Work out the finished part from the listing and answer in its coordinate system (mm). A direction names the side the tool comes from. Coordinates: 2 decimals unless noted, no trailing zeros. Order: outer loops, then holes, each group sorted by start corner. A loop starts at its lowest first (then second) coordinate and runs counter-clockwise, first axis right, second up.
Autodesk Inventor part; units mm, degrees
ref_plane "YZ Plane" through (0, 0, 0) normal (1, 0, 0) x (0, 1, 0)
ref_plane "XZ Plane" through (0, 0, 0) normal (0, 1, 0) x (-1, 0, 0)
ref_plane "XY Plane" through (0, 0, 0) normal (0, 0, 1) x (1, 0, 0)
sketch "Sketch1" plane through (0, 0, 0) normal (1, 0, 0) x (0, 1, 0)
  line L0 (0, 15) -> (2.5, 15) construction
  line L1 (0, 0) -> (9.4946, 0) construction
  arc A0 (9.4946, 0) -> (2.5, 15) centre (-10.0865, 0) ccw construction
  line L2 (0, 9.5) -> (0, 0) construction
  line L3 (9.4946, 0) -> (9, 0) construction
  line L4 (9, 0) -> (9, 15)
  line L5 (9, 15) -> (9, 15)
  line L6 (9, 15) -> (9, 17)
  line L7 (9, 17) -> (4.25, 17)
  line L8 (4.25, 17) -> (4.25, 15)
  line L9 (2.5, 15) -> (4.25, 15) construction
  line L10 (2.5, 15) -> (9.4946, 0) construction
  line L11 (3.25, 15) -> (3.25, 13.3916)
  line L12 (3.25, 15) -> (4.25, 15)
  line L13 (7.1631, 5) -> (7.1631, 0)
  line L14 (7.1631, 0) -> (9, 0)
  line L15 (7.1631, 5) -> (3.25, 13.3916)
  point P0 (2.25, 0)
  dimension "d2" = 15
  dimension "d12" = 2
  dimension "d14" = 0
  dimension "d16" = 2
  dimension "d17" = 4.25
  dimension "d35" = 115
  dimension "d36" = 9
  dimension "d37" = 2.5
  dimension "d39" = 1
  dimension "d40" = 5
  dimension "d41" = 7.1631
  dimension "d42" = 3.25
  dimension "d43" = 1.6084
  dimension "d44" = 8.3916
revolve "Revolution1" add sketch "Sketch1" angle 360 about axis through (0, 0, 9.5) along (0, 0, -1)
sketch "Sketch3" plane through (0, 0, 0) normal (1, 0, 0) x (0, 1, 0)
  line L0 (7.1631, 0) -> (14, 0)
  line L1 (14, 0) -> (14, 17)
  line L2 (14, 17) -> (7.1631, 17)
  line L3 (7.1631, 17) -> (7.1631, 0)
  line L4 (-7.1631, 0) -> (7.1631, 0) construction
  line L5 (-9, 17) -> (9, 17) construction
  point P0 (0, 0)
  dimension "d28" = 14
extrude "Extrusion1" add sketch "Sketch3" along normal mid plane 8
sketch "Sketch4" plane through (-4, 0, 0) normal (-1, 0, 0) x (0, 0, 1)
  circle A0 centre (5, 10.25) radius 1.6
  circle A1 centre (12, 10.25) radius 1.6
  line L0 (5, 10.25) -> (12, 10.25) construction
  line L1 (17, 14) -> (0, 14) construction
  point P0 (0, 0)
  point P1 (17, 10.25)
  point P2 (8.5, 10.25)
  point P3 (8.5, 14)
  dimension "d29" = 3.2
  dimension "d30" = 3.2
  dimension "d31" = 7
  dimension "d34" = 3.75
extrude "Extrusion2" cut sketch "Sketch4" against normal blind 10
properties part number "brush holder"
1. The part is cut by section A-A (y = 0). Determine the outline of the cut face in (x, z).
2. For faces 1 (the cylindrical face through (3.584, 2.285, 15.986)), 2 (the flat face through (-4, 11, 9)), 3 (the cylindrical face through (-0.1, 10.3, 10.4)), determine the directions among +Z, -Z, +X, -X, +Y, -Y from which every point of the face is accessible in a straight line to the end or side of a thin tool.
3. The mould has two halves that part along Y. Classify faces 4 (the flat face through (4, 11, 9)), 5 (the cylindrical face through (0, -9, 9)), 6 (the flat face through (0, 14, 8)), 7 (the cylindrical face through (2.152, 6.832, 2.465)): released by +Y, released by -Y, zero draft, split by the parting line, or undercut.
4. The part is cut by section B-B (x = 0). Determine the outline of the cut face in (y, z).
5. Consider probe 1 along X at (y, z) = (0, 3.6); probe 2 along Z at (x, y) = (-0.5, 10.5); probe 3 along Y at (x, z) = (-2, 5). Determine where each line is inside the solid, lowest interval first.
6. The part is cut by section D-D (z = 1.25). Determine the outline of the cut face in (x, y), plus the area to 3 significant figures.
7. Flat-ended cylindrical pins translate along their axes: pin 1 (10 mm diameter, centred on y = 3, z = 12.5, fed in from -X); pin 2 (5 mm diameter, centred on y = 10.25, z = 12, fed in from -X); pin 3 (5 mm diameter, centred on y = 10, z = 12.5, fed in from -X); pin 4 (5 mm diameter, centred on y = 12, z = 12.5, fed in from +X). Find the tip coordinate at first contact, or state that the pin passes through.
8. The part is cut by section C-C (z = 12). Determine the outline of the cut face in (x, y).
Worked out:
1. outline: (-9, 0) - (-7.16, 0) - (-7.16, 5) - (-3.25, 13.39) - (-3.25, 15) - (-4.25, 15) - (-4.25, 17) - (-9, 17) - close; (3.25, 13.39) - (7.16, 5) - (7.16, 0) - (9, 0) - (9, 17) - (4.25, 17) - (4.25, 15) - (3.25, 15) - close
2. face 1: +Z
2. face 2: +Z, -Z, -X, +Y
2. face 3: +X, -X
3. face 4: zero draft
3. face 5: split by the parting line
3. face 6: released by +Y
3. face 7: undercut
4. outline: (-9, 0) - (-7.16, 0) - (-7.16, 5) - (-3.25, 13.39) - (-3.25, 15) - (-4.25, 15) - (-4.25, 17) - (-9, 17) - close; (3.25, 13.39) - (7.16, 5) - (7.16, 0) - (14, 0) - (14, 17) - (4.25, 17) - (4.25, 15) - (3.25, 15) - close; hole circle Ø3.2 at (10.25, 5); hole circle Ø3.2 at (10.25, 12)
5. probe 1: x = -9 to -7.16, 7.16 to 9
5. probe 2: z = 0 to 3.42, 6.58 to 10.42, 13.58 to 17
5. probe 3: y = -8.77 to -6.88, 6.88 to 8.65, 11.85 to 14
6. outline: (-4, 8.06) arc R9 ccw (long way) to (4, 8.06) - (4, 14) - (-4, 14) - close; hole circle Ø14.33 at (0, 0)
6. area: 136 mm2
7. pin 1: stops at x = -9
7. pin 2: stops at x = -4.58
7. pin 3: stops at x = -4.97
7. pin 4: stops at x = 4
8. outline: (-4, 8.06) arc R9 ccw (long way) to (4, 8.06) - (4, 8.65) - (-4, 8.65) - close; (-4, 11.85) - (4, 11.85) - (4, 14) - (-4, 14) - close; hole circle Ø7.8 at (0, 0)
